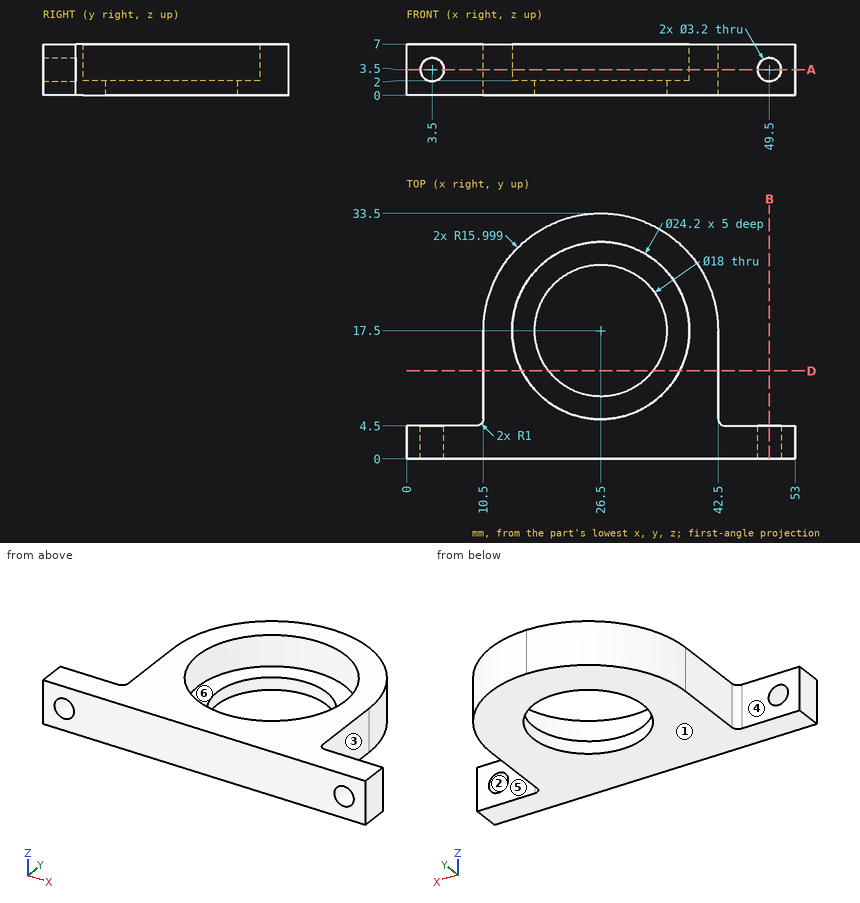
Answer from the drawing. Dimensions are ordinates in mm from the lowest x, y and z of the part. A direction names the side the tool comes from. Coordinates: 2 decimals unless noted, no trailing zeros. Order: outer loops, then holes, each group sorted by start corner. A loop starts at its lowest first (then second) coordinate and runs counter-clockwise, first axis right, second up. Notation, with made-up numbers: (-33.5, 0.25) - (-19.5, 0.25) arc R28 cw to (-19.5, 27.25) - close; hole circle Ø10 at (-7, 71.25). An arc over 180 degrees is marked (long way). Answer as a JSON object with one key per item and string values. Group by question number.
Item 1: Section B-B (x = 49.5) is taken. Give the vertices of the cut face in (y, z).
Item 2: Consider probe 1 along X at (y, z) = (1.9, 3.5); probe 2 along X at (y, z) = (17.5, 3.6); probe 3 along Z at (x, y) = (3.5, 1.5). Determine where each line is inside the solid, lowest interval first. Write a range as from..to.
Item 3: Section A-A (z = 3.5) is taken. State how many separate pieces and enclosed holes the cut face has.
Item 4: Section D-D (y = 12) is taken. Give the vertices of the cut face in (x, z).
Item 5: A tool of negligible diameter and unlimited length cuts with its end or side. For the marked faces 4, 5 and 6, from which of +Z, -Z, +X, -X, +Y, -Y can it reach the whole face along a straight path? Write none if from no direction.
Item 6: The mould has two halves that part along X. Classify the marked faces 1, 2 and 3: +X half, -X half, draft (parallel to the pull), parting line (faces both ways), or undercut.
Item 7: Flat-ended cylindrical pins translate along their axes: P1, Ø1, axis at y = 8, z = 2, coming from the -X side; P2, Ø7.5, axis at x = 30, y = 18.5, coming from the +Z side. Find the tip coordinate at first contact, or state that the pin passes through.
Results are:
{
 "1": {"outline": "(0, 0) - (4.5, 0) - (4.5, 1.9) - (0, 1.9) - close; (0, 5.1) - (4.5, 5.1) - (4.5, 7) - (0, 7) - close"},
 "2": {"probe 1": "x = 0..1.9, 5.1..47.9, 51.1..53", "probe 2": "x = 10.5..14.4, 38.6..42.5", "probe 3": "z = 0..1.9, 5.1..7"},
 "3": {"separate pieces": "3", "enclosed holes": "1"},
 "4": {"outline": "(10.5, 0) - (19.38, 0) - (19.38, 2) - (15.72, 2) - (15.72, 7) - (10.5, 7) - close; (33.62, 0) - (42.5, 0) - (42.5, 7) - (37.28, 7) - (37.28, 2) - (33.62, 2) - close"},
 "5": {"face 4": "+Z, -Z, -X, +Y", "face 5": "+Z, -Z, +X, +Y", "face 6": "+Z"},
 "6": {"face 1": "draft", "face 2": "undercut", "face 3": "+X half"},
 "7": {"P1": "stops at x = 10.5", "P2": "passes through"}
}
